```python
from build123d import *

# Parameters (mm, degrees)
BASE_FLANGE1_DEPTH  = 41
SKETCH2_R           = 2.5
CUT_EXTRUDE1_DEPTH  = 10
SKETCH3_R           = 2.75
SKETCH3_R_2         = 2.5
CUT_EXTRUDE2_DEPTH  = 10
BOSS_EXTRUDE1_START = -41
BOSS_EXTRUDE1_DEPTH = 41
SKETCH5_W           = 31.746142427
SKETCH5_H           = 33.611284957
CUT_EXTRUDE3_DEPTH  = 19
CUT_EXTRUDE4_START  = 2.688066512
CUT_EXTRUDE4_DEPTH  = 36.36668128
CUT_EXTRUDE5_DEPTH  = 3


# Read off the part's stored shape, not the designer's step: Cut-Extrude4, Cut-Extrude5
# Sheet-metal steps are written as plain solids
with BuildPart() as part:
    # Sketch1 → Base-Flange1 (new body)
    with BuildSketch(Plane(origin=(0, 0, 0), x_dir=(1, 0, 0), z_dir=(0, 1, 0))):
        with BuildLine():
            Line((0, 0), (29.484227127, 0))
            ThreePointArc((29.484227127, 0), (29.90672353, 0.133212604), (30.176404712, 0.484667962))
            Line((30.176404712, 0.484667962), (38.681704054, 23.85278585))
            ThreePointArc((38.681704054, 23.85278585), (40.049733788, 25.635636911), (42.1929595, 26.311393382))
            Line((42.1929595, 26.311393382), (78.441184331, 26.311393382))
            ThreePointArc((78.441184331, 26.311393382), (80.843024514, 25.437195048), (82.121016981, 23.223647163))
            Line((82.121016981, 23.223647163), (84.942198964, 7.223929074))
            ThreePointArc((84.942198964, 7.223929074), (85.194131001, 6.787569985), (85.667608355, 6.615238322))
            Line((85.667608355, 6.615238322), (158.049527566, 6.615238322))
            Line((158.049527566, 6.615238322), (158.049527566, 3.615238322))
            Line((158.049527566, 3.615238322), (85.667608355, 3.615238322))
            ThreePointArc((85.667608355, 3.615238322), (83.265768172, 4.489436656), (81.987775705, 6.702984541))
            Line((81.987775705, 6.702984541), (79.166593722, 22.70270263))
            ThreePointArc((79.166593722, 22.70270263), (78.914661685, 23.139061719), (78.441184331, 23.311393382))
            Line((78.441184331, 23.311393382), (42.1929595, 23.311393382))
            ThreePointArc((42.1929595, 23.311393382), (41.770463097, 23.178180778), (41.500781916, 22.82672542))
            Line((41.500781916, 22.82672542), (32.995482574, -0.541392468))
            ThreePointArc((32.995482574, -0.541392468), (31.627452839, -2.324243529), (29.484227127, -3))
            Line((29.484227127, -3), (0, -3))
            Line((0, -3), (0, 0))
        make_face()
    extrude(amount=BASE_FLANGE1_DEPTH)

    # Sketch2 → Cut-Extrude1 (cut)
    with BuildSketch(Plane.XY.offset(3)):
        with Locations((14.991664351, 20)):
            Circle(SKETCH2_R)
    extrude(amount=-CUT_EXTRUDE1_DEPTH, mode=Mode.SUBTRACT)

    # Sketch3 → Cut-Extrude2 (cut)
    with BuildSketch(Plane.XY.offset(-3.615238322)):
        with Locations((134.991664351, 21)):
            Circle(SKETCH3_R)
        with Locations((14.991664351, 20)):
            Circle(SKETCH3_R_2)
    extrude(amount=-CUT_EXTRUDE2_DEPTH, mode=Mode.SUBTRACT)

    # Sketch4 → Boss-Extrude1 (add)
    with BuildSketch(Plane(origin=(0, 41, 0), x_dir=(1, 0, 0), z_dir=(0, 1, 0)).offset(BOSS_EXTRUDE1_START)):
        with BuildLine():
            Line((29.484227127, -3), (75.654085032, -3))
            ThreePointArc((75.654085032, -3), (82.030907409, -1.766249423), (85.667608355, 3.615238322))
            ThreePointArc((85.667608355, 3.615238322), (83.265768172, 4.489436656), (81.987775705, 6.702984541))
            ThreePointArc((81.987775705, 6.702984541), (80.181574687, 2.106348284), (75.654085032, 0.133212604))
            Line((75.654085032, 0.133212604), (29.90672353, 0.133212604))
            Line((29.90672353, 0.133212604), (29.484227127, -3))
        make_face()
    extrude(amount=BOSS_EXTRUDE1_DEPTH)

    # Sketch5 → Cut-Extrude3 (cut)
    with BuildSketch(Plane.XY.offset(-23.311393382)):
        with Locations((60.358708807, 21.215436548)):
            Rectangle(SKETCH5_W, SKETCH5_H)
    extrude(amount=-CUT_EXTRUDE3_DEPTH, mode=Mode.SUBTRACT)

    # Cut-Extrude4 outline → Cut-Extrude4 (cut)
    with BuildSketch(Plane(origin=(0, 0, 0), x_dir=(1, 0, 0), z_dir=(0, 1, 0)).offset(CUT_EXTRUDE4_START)):
        Polygon((79.368642173, 21.556828923), (81.806889388, 7.728841823), (84.761312647, 8.249786356), (82.323065432, 22.077773456), align=None)
        Polygon((38.219499528, 22.582889353), (33.376132128, 9.275846786), (36.19520999, 8.249786356), (41.038577391, 21.556828923), align=None)
    extrude(amount=CUT_EXTRUDE4_DEPTH, mode=Mode.SUBTRACT)

    # Cut-Extrude5 outline → Cut-Extrude5 (cut)
    with BuildSketch(Plane.XY):
        with BuildLine():
            Line((0, 41), (0, 35.818729295))
            ThreePointArc((0, 35.818729295), (1.526422616, 39.473577384), (5.181270705, 41))
            Line((5.181270705, 41), (0, 41))
        make_face()
        with BuildLine():
            ThreePointArc((5.188265578, 0), (1.627560559, 1.417661865), (0, 4.887450335))
            Line((0, 4.887450335), (0, 0))
            Line((0, 0), (5.188265578, 0))
        make_face()
    extrude(amount=CUT_EXTRUDE5_DEPTH, mode=Mode.SUBTRACT)


solid = part.part
```
Can you work these out from the model? Positions are in its coordinate system, mm. A direction names the side the tool comes from. Give positions to 0.01 mm unless a question says otherwise; leave off trailing zeros. Loops run counter-clockwise (first coordinate to the right, second up) from the corner with the lowest first, then second, coordinate; pieces in that order, holes last. Notation, with made-up numbers: M 33,41 L 73,41 A20 cw 73,62 Z; hole C 35,16.25 d6. An arc over 180 degrees is marked long. One line per item, written item: value.
(1) Suppose I cut it at A-A on x = 46. List the corners of the cut face in (y, z) for me, plus the area to 3 significant figures.
Returned:
outline: M 0,-26.31 L 4.41,-26.31 L 4.41,-23.31 L 0,-23.31 Z; M 0,-0.13 L 41,-0.13 L 41,3 L 0,3 Z; M 38.02,-26.31 L 41,-26.31 L 41,-23.31 L 38.02,-23.31 Z
area: 151 mm^2
(2) Suppose I cut it at D-D on x = 134. List the corners of the cut face in (y, z) for me.
Returned:
outline: M 0,-6.62 L 18.44,-6.62 L 18.44,-3.62 L 0,-3.62 Z; M 23.56,-6.62 L 41,-6.62 L 41,-3.62 L 23.56,-3.62 Z
(3) We'd pull the mould along Y, two halves only. Please class faces 5 (the face through (81.3, 0, -11.6)), 6 (the face through (44.486, 21, -25)), 7 (the face through (77, 20, -23.311)): released by +Y, released by -Y, zero draft, split by the parting line, or undercut.
Returned:
face 5: released by -Y
face 6: undercut
face 7: zero draft
(4) I need wall thicknesses on line 1 (Z direction, x = 18, y = 31); line 2 (Z direction, x = 95, y = 38); line 3 (X direction, y = 17, z = -3). Which ranges of each line are inside material? Lowest first, please.
Returned:
line 1: 0 to 3
line 2: -6.62 to -3.62
line 3: 31.09 to 34.28, 80.9 to 85.52
(5) Suppose I cut it at B-B on y = 27.5. Count the separate pieces of the cut face and the enclosed holes in it, plus the area to 3 significant figures.
Returned:
separate pieces: 3
enclosed holes: 0
area: 572 mm^2
(6) Which directions (+Z, -Z, +X, -X, +Y, -Y) give clear straight access to the entire face, cutting with the end or side of a thin tool? Please do faces 1 (the face through (39.649, 20.617, -22.063)), 2 (the face through (76.232, 21, -25)), 3 (the face through (80.23, 20.21, -2.16)), 4 (the face through (121, 20, -6.615)).
Returned:
face 1: -X
face 2: -Z
face 3: +Y, -Y
face 4: -Z, +X, +Y, -Y
(7) Suppose I cut it at C-C on z = -14. List the corners of the cut face in (x, y) for me, plus the area to 3 significant figures.
Returned:
outline: M 35.1,0 L 38.29,0 L 38.29,2.69 L 35.1,2.69 Z; M 35.1,39.05 L 38.29,39.05 L 38.29,41 L 35.1,41 Z; M 80.7,0 L 83.75,0 L 83.75,2.69 L 80.7,2.69 Z; M 80.7,39.05 L 83.75,39.05 L 83.75,41 L 80.7,41 Z
area: 28.9 mm^2
(8) Will these pins go through, and if not, where does the flat tip stop? pin 1 (2 mm diameter, centred on x = 81.5, y = 6, fed in from -Z); pin 2 (6 mm diameter, centred on x = 33, y = 18, fed in from +Z); pin 3 (4.5 mm diameter, centred on x = 134.99, y = 21, fed in from +Z); pin 4 (8 mm diameter, centred on x = 140, y = 9, fed in from -Z).
Returned:
pin 1: z = -25.69
pin 2: z = 3
pin 3: through
pin 4: z = -6.62
